from build123d import *

# Parameters (mm, degrees)
BOSS_EXTRUDE1_DEPTH     = 5
SKETCH4_W               = 50
SKETCH4_H               = 50
BOSS_EXTRUDE2_DEPTH     = 30
CUT_EXTRUDE1_DEPTH      = 25
CUT_EXTRUDE2_DEPTH      = 50.749371855
CUT_EXTRUDE2_DEPTH_BACK = 50.749371855
CUT_EXTRUDE3_DEPTH      = 50.749371855
CUT_EXTRUDE3_DEPTH_BACK = 50.749371855
SKETCH7_W               = 50
SKETCH7_H               = 50
FILLET2_R               = 1
CHAMFER1_SIZE           = 0.5


with BuildPart() as part:
    # Sketch3 → Boss-Extrude1 (new body)
    with BuildSketch(Plane(origin=(0, 0, 0), x_dir=(1, 0, 0), z_dir=(0, 1, 0))):
        Polygon((14.43375673, 0), (7.216878365, 12.5), (-7.216878365, 12.5), (-14.43375673, 0), (-7.216878365, -12.5), (7.216878365, -12.5), align=None)
    extrude(amount=BOSS_EXTRUDE1_DEPTH)

    # Sketch4 → Boss-Extrude2 (add)
    with BuildSketch(Plane(origin=(0, 5, 0), x_dir=(1, 0, 0), z_dir=(0, 1, 0))):
        Rectangle(SKETCH4_W, SKETCH4_H)
    extrude(amount=BOSS_EXTRUDE2_DEPTH)

    # Sketch5 → Cut-Extrude1 (cut)
    with BuildSketch(Plane(origin=(0, 35, 0), x_dir=(1, 0, 0), z_dir=(0, 1, 0))):
        Polygon((0, 15.877132403), (-13.75, 7.938566201), (-13.75, -7.938566201), (0, -15.877132403), (13.75, -7.938566201), (13.75, 7.938566201), align=None)
    extrude(amount=-CUT_EXTRUDE1_DEPTH, mode=Mode.SUBTRACT)

    # Sketch6 → Cut-Extrude2 (cut, two sides: drawn at the far end of the back side and taken through both)
    with BuildSketch(Plane.XZ.offset(-CUT_EXTRUDE2_DEPTH_BACK)):
        Polygon((-12.124355653, 0), (-6.062177826, -10.5), (6.062177826, -10.5), (12.124355653, 0), (6.062177826, 10.5), (-6.062177826, 10.5), align=None)
    extrude(amount=CUT_EXTRUDE2_DEPTH + CUT_EXTRUDE2_DEPTH_BACK, mode=Mode.SUBTRACT)

    # Sketch7 → Cut-Extrude3 (cut, two sides: drawn at the far end of the back side and taken through both)
    with BuildSketch(Plane(origin=(0, 35, 0), x_dir=(1, 0, 0), z_dir=(0, 1, 0)).offset(-CUT_EXTRUDE3_DEPTH_BACK)):
        Rectangle(SKETCH7_W, SKETCH7_H)
        Polygon((-23.405444566, 5.539419162), (6.905444566, 23.039419162), (23.405444566, -5.539419162), (-6.905444566, -23.039419162), align=None, mode=Mode.SUBTRACT)
    extrude(amount=CUT_EXTRUDE3_DEPTH + CUT_EXTRUDE3_DEPTH_BACK, mode=Mode.SUBTRACT)

    # Fillet2
    fillet2_edges = [part.edges().sort_by_distance(p)[0] for p in [
        (-15.155444566, 5, 8.75),
        (-8.25, 5, -14.289419162),
        (15.155444566, 5, -8.75),
        (8.25, 5, 14.289419162),
        (-23.405444566, 20, -5.539419162),
        (-15.155444566, 35, 8.75),
        (6.905444566, 20, -23.039419162),
        (-8.25, 35, -14.289419162),
        (23.405444566, 20, 5.539419162),
        (15.155444566, 35, -8.75),
        (-6.905444566, 20, 23.039419162),
        (8.25, 35, 14.289419162),
    ]]
    fillet(fillet2_edges, radius=FILLET2_R)

    # Chamfer1
    chamfer1_edges = [part.edges().sort_by_distance(p)[0] for p in [
        (6.875, 35, -11.907849302),
        (-6.875, 35, -11.907849302),
        (-13.75, 35, 0),
        (-6.875, 35, 11.907849302),
        (6.875, 35, 11.907849302),
        (13.75, 35, 0),
    ]]
    chamfer(chamfer1_edges, length=CHAMFER1_SIZE)


solid = part.part
Geometry: final body of the model. Coordinates: model frame, mm. A direction names the side the tool comes from. Round coordinates to 2 decimals unless told otherwise and drop trailing zeros. Loops run counter-clockwise (first coordinate to the right, second up) from the corner with the lowest first, then second, coordinate; pieces in that order, holes last. Notation, with made-up numbers: (-7.5, 11) - (2.5, 11) arc R18 ccw to (2.5, 42) - close; hole circle Ø10 at (49, -10.5). An arc over 180 degrees is marked (long way). Write each question's results on one line, items separated by ' | '. Start each with the question number.
1) Cut plane A-A on y = 8.5. Return loops of the section in (x, z), then the cut area to 3 significant figures.
2) First-contact query: P1, Ø8, axis at x = -1.5, y = 7, coming from the +Z side; P2, Ø5, axis at x = -1, y = 3, coming from the -Z side; P3, Ø5.5, axis at x = 3, y = 2.5, coming from the +Z side; P4, Ø1.5, axis at x = 6, z = 8, coming from the +Y side. Flat tips, straight axial feed; report the tip coordinate or a pass-through.
3) Access query for faces 1 (the face through (-9.051, 5.07, 5.324)), 2 (the face through (-7.098, 34.747, 12.064)), 3 (the face through (-2, 5, 13)), 4 (the face through (14.79, 5.29, -8.79)), 5 (the face through (-10.775, 2.465, -6.337)). Directions: +Z, -Z, +X, -X, +Y, -Y. A direction counts if a zero-diameter tool reaches every point of the face in a straight line with its end or side. Return the directions, or none.
4) Mould query, pull axis X, two halves, no side actions, for faces 6 (the face through (-6.971, 22.422, 11.852)), 7 (the face through (10, 0, 5)), 8 (the face through (-13.75, 22, 0)), 9 (the face through (23.01, 20.2, 5.42)). Classes: released by +X, released by -X, zero draft, split by the parting line, or undercut.
5) Cut plane B-B on y = 14.5. Return loops of the section in (x, z), then the cut area to 3 significant figures.
6) Line query: probe 1 along Y at (x, z) = (0, -15); probe 2 along Z at (x, y) = (-12, 2); probe 3 along Z at (x, y) = (1, 26.5). Output: solid intervals per line, ascending. Write a range as [from, to].
Verdict:
1) outline: (-22.91, -4.67) arc R1 ccw to (-22.54, -6.04) - (6.04, -22.54) arc R1 ccw to (7.41, -22.17) - (22.91, 4.67) arc R1 ccw to (22.54, 6.04) - (-6.04, 22.54) arc R1 ccw to (-7.41, 22.17) - close; hole (-12.12, 0) - (-6.06, -10.5) - (6.06, -10.5) - (12.12, 0) - (6.06, 10.5) - (-6.06, 10.5) - close | area: 772 mm2
2) P1: stops at z = 22.23 | P2: stops at z = -18.71 | P3: stops at z = 17.2 | P4: passes through
3) face 1: +Y, -Y | face 2: +Y | face 3: -Y | face 4: -Z, +X, -Y | face 5: -Z, -X, -Y
4) face 6: undercut | face 7: zero draft | face 8: undercut | face 9: released by +X
5) outline: (-22.91, -4.67) arc R1 ccw to (-22.54, -6.04) - (6.04, -22.54) arc R1 ccw to (7.41, -22.17) - (22.91, 4.67) arc R1 ccw to (22.54, 6.04) - (-6.04, 22.54) arc R1 ccw to (-7.41, 22.17) - close; hole (-13.75, -7.94) - (0, -15.88) - (13.75, -7.94) - (13.75, 7.94) - (0, 15.88) - (-13.75, 7.94) - close | area: 499 mm2
6) probe 1: y = [5, 10] | probe 2: z = [-4.22, -0.22], [0.22, 4.22] | probe 3: z = [-19.63, -15.3], [15.3, 18.48]
